from build123d import *

# Parameters (mm, degrees)
SKETCH1_W           = 50.8
SKETCH1_H           = 25.4
SKETCH1_W_2         = 44.45
SKETCH1_H_2         = 19.05
BOSS_EXTRUDE1_DEPTH = 692.15
SKETCH2_W           = 60.325
SKETCH2_H           = 12.7
CUT_EXTRUDE1_DEPTH  = 695.127907882
SKETCH3_R           = 3.175
CUT_EXTRUDE2_DEPTH  = 695.127907882
SKETCH4_W           = 12.7
SKETCH4_H           = 4.7625
CUT_EXTRUDE3_DEPTH  = 695.127907882
SKETCH5_R           = 3.175
SKETCH5_R_2         = 2.0828
CUT_EXTRUDE4_DEPTH  = 694.081483305
CUT_EXTRUDE5_DEPTH  = 3.175
SKETCH8_R           = 3.175
CUT_EXTRUDE6_DEPTH  = 694.081483305


with BuildPart() as part:
    # Sketch1 → Boss-Extrude1 (new body)
    with BuildSketch(Plane.XY):
        Rectangle(SKETCH1_W, SKETCH1_H)
        Rectangle(SKETCH1_W_2, SKETCH1_H_2, mode=Mode.SUBTRACT)
    extrude(amount=BOSS_EXTRUDE1_DEPTH)

    # Sketch2 → Cut-Extrude1 (cut, through all)
    with BuildSketch(Plane(origin=(25.4, 0, 0), x_dir=(0, 0, -1), z_dir=(1, 0, 0))):
        with Locations((-131.7625, 6.35)):
            Rectangle(SKETCH2_W, SKETCH2_H)
    extrude(amount=-CUT_EXTRUDE1_DEPTH, mode=Mode.SUBTRACT)

    # Sketch3 → Cut-Extrude2 (cut, through all)
    with BuildSketch(Plane(origin=(25.4, 0, 0), x_dir=(0, 0, -1), z_dir=(1, 0, 0))):
        with Locations((-167.999918, 0)):
            Circle(SKETCH3_R)
        with Locations((-91.813888, 0)):
            Circle(SKETCH3_R)
    extrude(amount=-CUT_EXTRUDE2_DEPTH, mode=Mode.SUBTRACT)

    # Sketch4 → Cut-Extrude3 (cut, through all)
    with BuildSketch(Plane(origin=(25.4, 0, 0), x_dir=(0, 0, -1), z_dir=(1, 0, 0))):
        with Locations((-168.275, 10.31875)):
            Rectangle(SKETCH4_W, SKETCH4_H)
    extrude(amount=-CUT_EXTRUDE3_DEPTH, mode=Mode.SUBTRACT)

    # Sketch5 → Cut-Extrude4 (cut, through all)
    with BuildSketch(Plane(origin=(0, 12.7, 0), x_dir=(1, 0, 0), z_dir=(0, 1, 0))):
        with Locations(Location((0, -207.85963, 0), (0, 0, 180))):
            Circle(SKETCH5_R)
        with Locations(Location((0, -365.440722, 0), (0, 0, 180))):
            Circle(SKETCH5_R)
        with Locations(Location((0, -413.111442, 0), (0, 0, 180))):
            Circle(SKETCH5_R)
        with Locations(Location((0, -452.759064, 0), (0, 0, 180))):
            Circle(SKETCH5_R)
        with Locations(Location((-12.7, -478.159064, 0), (0, 0, 180))):
            Circle(SKETCH5_R)
        with Locations(Location((12.7, -478.159064, 0), (0, 0, 180))):
            Circle(SKETCH5_R)
        with Locations(Location((-12.7, -579.759064, 0), (0, 0, 180))):
            Circle(SKETCH5_R)
        with Locations(Location((12.7, -579.759064, 0), (0, 0, 180))):
            Circle(SKETCH5_R)
        with Locations(Location((0, -605.159064, 0), (0, 0, 180))):
            Circle(SKETCH5_R)
        with Locations(Location((-12.7, -644.806686, 0), (0, 0, 180))):
            Circle(SKETCH5_R)
        with Locations(Location((12.7, -644.806686, 0), (0, 0, 180))):
            Circle(SKETCH5_R)
        with Locations(Location((0, -684.454308, 0), (0, 0, 180))):
            Circle(SKETCH5_R)
        with Locations(Location((0, -548.009064, 0), (0, 0, 180))):
            Circle(SKETCH5_R_2)
        with Locations(Location((0, -535.309064, 0), (0, 0, 180))):
            Circle(SKETCH5_R_2)
        with Locations(Location((0, -522.609064, 0), (0, 0, 180))):
            Circle(SKETCH5_R_2)
        with Locations(Location((0, -509.909064, 0), (0, 0, 180))):
            Circle(SKETCH5_R_2)
    extrude(amount=-CUT_EXTRUDE4_DEPTH, mode=Mode.SUBTRACT)

    # Sketch7 → Cut-Extrude5 (cut)
    with BuildSketch(Plane(origin=(0, 12.7, 0), x_dir=(1, 0, 0), z_dir=(0, 1, 0))):
        with BuildLine():
            Line((-12.7, -548.009064), (-12.7, -509.909064))
            ThreePointArc((-12.7, -509.909064), (0, -497.209064), (12.7, -509.909064))
            Line((12.7, -509.909064), (12.7, -548.009064))
            ThreePointArc((12.7, -548.009064), (0, -560.709064), (-12.7, -548.009064))
        make_face()
    extrude(amount=-CUT_EXTRUDE5_DEPTH, mode=Mode.SUBTRACT)

    # Sketch8 → Cut-Extrude6 (cut, through all)
    with BuildSketch(Plane(origin=(0, 12.7, 0), x_dir=(1, 0, 0), z_dir=(0, 1, 0))):
        with Locations(Location((0, -12.7, 0), (0, 0, 180))):
            Circle(SKETCH8_R)
        with Locations(Location((0, -38.1, 0), (0, 0, 180))):
            Circle(SKETCH8_R)
        with Locations(Location((0, -63.5, 0), (0, 0, 180))):
            Circle(SKETCH8_R)
    extrude(amount=-CUT_EXTRUDE6_DEPTH, mode=Mode.SUBTRACT)


solid = part.part
The listing builds one solid part. Answer for the finished solid, in the listing's coordinates (mm). A direction names the side the tool comes from. Give positions to 0.01 mm unless a question says otherwise; leave off trailing zeros. Write each loop counter-clockwise with the first axis right and the second up, starting at its lowest first coordinate (ties: lowest second). Pieces come first, ordered by that corner, then holes. Notation, with made-up numbers: (7.25, -19.5) -> (12.25, -19.5) arc R18 ccw to (12.25, 1.5) -> close; hole circle Ø2 at (85.5, 78.25). An arc over 180 degrees is marked (long way). Use a Markdown table: item, result.
(1) Find the intervals of material crossed by probe 1 along Z at (x, y) = (13, 10) (3 decimals); probe 2 along Z at (x, y) = (22.5, 0.75) (3 decimals); probe 3 along X at (y, z) = (6.25, 178) (3 decimals), in increasing order. Write a range as from..to.
Return value:
| item | result |
|---|---|
| probe 1 | 0..101.6, 174.625..474.998, 481.32..576.598, 582.92..641.646, 647.967..692.15 |
| probe 2 | 0..88.729, 94.899..101.6, 161.925..164.915, 171.085..692.15 |
| probe 3 | -25.4..-22.225, 22.225..25.4 |
(2) For faces 1 (the cylindrical face through (0.279, 11.135, 560.706)), 2 (the flat face through (0, 10, 101.6)), 3 (the flat face through (0, 9.525, 430)), determine the directions among +Z, -Z, +X, -X, +Y, -Y from which every point of the face is accessible in a straight line to the end or side of a thin tool.
Return value:
| item | result |
|---|---|
| face 1 | +Y |
| face 2 | +X, -X, +Y |
| face 3 | +Z, -Z |
(3) Determine the mould class of faces 4 (the flat face through (-25.4, 0, 341)), 5 (the flat face through (22.225, 0, 341)), 6 (the flat face through (0, 12.7, 50)), 7 (the cylindrical face through (-0.279, 11.135, 497.212)) for opening direction X: released by +X, released by -X, zero draft, split by the parting line, or undercut.
Return value:
| item | result |
|---|---|
| face 4 | released by -X |
| face 5 | undercut |
| face 6 | zero draft |
| face 7 | undercut |
(4) Flat-ended cylindrical pins translate along their axes: P1, Ø2.5, axis at x = -23.5, z = 143, coming from the +Y side; P2, Ø1.6, axis at x = 23.5, z = 168.5, coming from the +Y side. Find the tip coordinate at first contact, or state that the pin passes through.
Return value:
| item | result |
|---|---|
| P1 | y = 0 |
| P2 | y = 7.94 |
(5) Section A-A, the plane z = 295.5 is taken. Determine the outline of the cut face in (x, y) (3 decimals).
Return value:
| item | result |
|---|---|
| outline | (-25.4, -12.7) -> (25.4, -12.7) -> (25.4, 12.7) -> (-25.4, 12.7) -> close; hole (-22.225, -9.525) -> (22.225, -9.525) -> (22.225, 9.525) -> (-22.225, 9.525) -> close |
